from build123d import *

# Parameters (mm, degrees)
SKETCH1_R           = 200
BOSS_EXTRUDE1_DEPTH = 10
SKETCH2_R           = 22.5
CUT_EXTRUDE1_DEPTH  = 10
SKETCH3_R           = 6
CUT_EXTRUDE2_DEPTH  = 10
CIRPATTERN1_COUNT   = 16
SKETCH4_R           = 6
CUT_EXTRUDE3_DEPTH  = 10
CIRPATTERN2_COUNT   = 16


with BuildPart() as part:
    # Sketch1 → Boss-Extrude1 (new body)
    with BuildSketch(Plane(origin=(0, 0, 0), x_dir=(0, 0, -1), z_dir=(1, 0, 0))):
        Circle(SKETCH1_R)
    extrude(amount=BOSS_EXTRUDE1_DEPTH)

    # Sketch2 → Cut-Extrude1 (cut)
    with BuildSketch(Plane(origin=(10, 0, 0), x_dir=(0, 0, -1), z_dir=(1, 0, 0))):
        Circle(SKETCH2_R)
    extrude(amount=-CUT_EXTRUDE1_DEPTH, mode=Mode.SUBTRACT)

    # Sketch3 → Cut-Extrude2 (cut)
    with BuildSketch(Plane(origin=(10, 0, 0), x_dir=(0, 0, -1), z_dir=(1, 0, 0))):
        with Locations((110, 0)):
            Circle(SKETCH3_R)
    cut_extrude2 = extrude(amount=-CUT_EXTRUDE2_DEPTH, mode=Mode.SUBTRACT)

    # CirPattern1: Cut-Extrude2 ×16 about axis
    cirpattern1_axis = Axis((0, 0, 0), (1, 0, 0))
    for i in range(1, CIRPATTERN1_COUNT):
        add(cut_extrude2.rotate(cirpattern1_axis, i * 360 / CIRPATTERN1_COUNT), mode=Mode.SUBTRACT)

    # Sketch4 → Cut-Extrude3 (cut)
    with BuildSketch(Plane(origin=(10, 0, 0), x_dir=(0, 0, -1), z_dir=(1, 0, 0))):
        with Locations((180, 0)):
            Circle(SKETCH4_R)
    cut_extrude3 = extrude(amount=-CUT_EXTRUDE3_DEPTH, mode=Mode.SUBTRACT)

    # CirPattern2: Cut-Extrude3 ×16 about axis
    cirpattern2_axis = Axis((0, 0, 0), (1, 0, 0))
    for i in range(1, CIRPATTERN2_COUNT):
        add(cut_extrude3.rotate(cirpattern2_axis, i * 360 / CIRPATTERN2_COUNT), mode=Mode.SUBTRACT)


solid = part.part
Work out the finished part from the listing and answer in its coordinate system (mm). Give positions to 0.01 mm unless a question says otherwise; leave off trailing zeros. Order: outer loops, then holes, each group sorted by start corner. A loop starts at its lowest first (then second) coordinate and runs counter-clockwise, first axis right, second up. Notation, with made-up numbers: (70.25, -31.75) -> (100.25, -31.75) arc R19 cw to (100.25, -11.75) -> close; hole circle Ø2 at (-9, 74). An arc over 180 degrees is marked (long way). Answer as a JSON object with one key per item and string values. Group by question number.
1. Section D-D on z = 150.5 is taken. Determine the outline of the cut face in (x, y), plus the area to 3 significant figures.
2. Section B-B on x = 8 is taken. Count the separate pieces of the cut face and the enclosed holes in it, plus the area to 3 significant figures.
3. Section C-C on z = -148 is taken. Determine the outline of the cut face in (x, y).
4. Flat-ended cylindrical pins translate along their axes: pin 1 Ø5 at (x, z) = (5, 58) entering from +Y; pin 2 Ø3 at (x, z) = (5, 37) entering from -Y; pin 3 Ø3 at (x, z) = (1, -122) entering from -Y. Find the tip coordinate at first contact, or state that the pin passes through.
5. Consider line 1 along Z through (x, y) = (3.25, -162); line 2 along Z through (x, y) = (9.25, -5); line 3 along Y through (x, z) = (1.75, -171). Determine where each line is inside the solid, lowest interval first. Write a range as [from, to].
6. Section A-A on y = 180 is taken. Determine the outline of the cut face in (x, z), plus the area to 3 significant figures.
Result sheet:
{
 "1": {"outline": "(0, -131.72) -> (10, -131.72) -> (10, 131.72) -> (0, 131.72) -> close", "area": "2,630 mm^2"},
 "2": {"separate pieces": "1", "enclosed holes": "33", "area": "120,000 mm^2"},
 "3": {"outline": "(0, -134.52) -> (10, -134.52) -> (10, 134.52) -> (0, 134.52) -> close"},
 "4": {"pin 1": "stops at y = 192.15", "pin 2": "stops at y = -196.82", "pin 3": "stops at y = -159.62"},
 "5": {"line 1": "z = [-117.29, -73.07], [-64.7, 64.7], [73.07, 117.29]", "line 2": "z = [-199.94, -183.32], [-176.68, -113.32], [-106.68, -21.94], [21.94, 106.68], [113.32, 176.68], [183.32, 199.94]", "line 3": "y = [-103.73, -72.61], [-65.16, 65.16], [72.61, 103.73]"},
 "6": {"outline": "(0, -87.18) -> (10, -87.18) -> (10, -6) -> (0, -6) -> close; (0, 6) -> (10, 6) -> (10, 87.18) -> (0, 87.18) -> close", "area": "1,620 mm^2"}
}
